```python
from build123d import *

# Parameters (mm, degrees)
SKETCH_1_R      = 2
SKETCH_1_R_2    = 1
EXTRUDE_1_DEPTH = 2
FILLET_1_R      = 2


with BuildPart() as part:
    # 草图1 → 凸台-拉伸1 (new body)
    with BuildSketch(Plane.XY):
        with BuildLine():
            Line((41.276428571, -8.854285714), (-42.723571429, -8.854285714))
            Line((-42.723571429, -8.854285714), (-42.723571429, -21.854285714))
            Line((-42.723571429, -21.854285714), (-54.723571429, -21.854285714))
            Line((-54.723571429, -21.854285714), (-54.723571429, 22.145714286))
            Line((-54.723571429, 22.145714286), (-42.723571429, 22.145714286))
            Line((-42.723571429, 22.145714286), (-42.723571429, 9.145714286))
            Line((-42.723571429, 9.145714286), (41.276428571, 9.145714286))
            ThreePointArc((41.276428571, 9.145714286), (50.276428571, 0.145714286), (41.276428571, -8.854285714))
        make_face()
        with Locations((1.276428571, 0.145714286)):
            Circle(SKETCH_1_R, mode=Mode.SUBTRACT)
        with Locations((-48.723571429, 16.645714286)):
            Circle(SKETCH_1_R, mode=Mode.SUBTRACT)
        with Locations((-48.723571429, -16.354285714)):
            Circle(SKETCH_1_R, mode=Mode.SUBTRACT)
        with Locations((41.276428571, 6.145714286)):
            Circle(SKETCH_1_R_2, mode=Mode.SUBTRACT)
        with Locations((47.276428571, 0.145714286)):
            Circle(SKETCH_1_R_2, mode=Mode.SUBTRACT)
        with Locations((41.276428571, -5.854285714)):
            Circle(SKETCH_1_R_2, mode=Mode.SUBTRACT)
        with Locations((35.276428571, 0.145714286)):
            Circle(SKETCH_1_R_2, mode=Mode.SUBTRACT)
    extrude(amount=EXTRUDE_1_DEPTH)

    # 圆角1
    fillet_1_edges = [part.edges().sort_by_distance(p)[0] for p in [
        (-42.723571429, -8.854285714, 1),
        (-42.723571429, -21.854285714, 1),
        (-54.723571429, -21.854285714, 1),
        (-54.723571429, 22.145714286, 1),
        (-42.723571429, 22.145714286, 1),
        (-42.723571429, 9.145714286, 1),
    ]]
    fillet(fillet_1_edges, radius=FILLET_1_R)


solid = part.part
```
Can you work these out from the model? Positions are in its coordinate system, mm. A direction names the side the tool comes from. Round coordinates to 2 decimals unless told otherwise and drop trailing zeros. Loops run counter-clockwise (first coordinate to the right, second up) from the corner with the lowest first, then second, coordinate; pieces in that order, holes last.
Item 1: Which directions (+Z, -Z, +X, -X, +Y, -Y) give clear straight access to the entire face, cutting with the end or side of a thin tool? Please do faces 5 (the cylindrical face through (-42.12, -9.42, 1.01)), 6 (the flat face through (0, 9.146, 1)).
Item 2: Suppose I cut it at B-B, the plane x = 2. Write out the boundary of the cut face in (y, z), then the cut area to 3 significant figures.
Item 3: Please list where these lines run through material, in increasing order: L1, parallel to X at y = 0, z = 1.6; L2, parallel to X at y = 1, z = 1.65; L3, parallel to Y at x = -6.5, z = 0.9.
Item 4: Will this pin go through, and if not, where does the flat tip stop? pin 1 Ø1 at (x, z) = (-6.5, 1) entering from -Y.
Item 5: Suppose I cut it at C-C, the plane x = 23.5. Write out the boundary of the cut face in (y, z), then the cut area to 3 significant figures.
Item 6: Suppose I cut it at D-D, the plane y = 13. Write out the boundary of the cut face in (x, z).
Item 7: If we mould it in two halves opening along Y, with no side actions, what happens to faces 1 (the flat face through (-13, 0, 2)), 2 (the cylindrical face through (-43.29, 21.54, 1.01)), 3 (the cylindrical face through (42.23, 6.45, 0.99)), 4 (the flat face through (1, -8.854, 1))? For each: +Y half, -Y half, draft (parallel to the pull), parting line (faces both ways), or undercut.
Item 8: Suppose I cut it at A-A, the plane z = 1.1. Write out the boundary of the cut face in (x, y).
Reported:
1. face 5: +Z, -Z, +X, -Y
1. face 6: +Z, -Z, +X, +Y
2. outline: (-8.85, 0) - (-1.72, 0) - (-1.72, 2) - (-8.85, 2) - close; (2.01, 0) - (9.15, 0) - (9.15, 2) - (2.01, 2) - close
2. area: 28.5 mm2
3. L1: x = -54.72 to -0.72, 3.27 to 34.29, 36.27 to 46.29, 48.27 to 50.28
3. L2: x = -54.72 to -0.53, 3.08 to 34.76, 35.8 to 46.76, 47.8 to 50.24
3. L3: y = -8.85 to 9.15
4. pin 1: stops at y = -8.85
5. outline: (-8.85, 0) - (9.15, 0) - (9.15, 2) - (-8.85, 2) - close
5. area: 36.0 mm2
6. outline: (-54.72, 0) - (-42.72, 0) - (-42.72, 2) - (-54.72, 2) - close
7. face 1: draft
7. face 2: +Y half
7. face 3: undercut
7. face 4: -Y half
8. outline: (-54.72, -19.85) arc R2 ccw to (-52.72, -21.85) - (-44.72, -21.85) arc R2 ccw to (-42.72, -19.85) - (-42.72, -10.85) arc R2 cw to (-40.72, -8.85) - (41.28, -8.85) arc R9 ccw to (41.28, 9.15) - (-40.72, 9.15) arc R2 cw to (-42.72, 11.15) - (-42.72, 20.15) arc R2 ccw to (-44.72, 22.15) - (-52.72, 22.15) arc R2 ccw to (-54.72, 20.15) - close; hole circle Ø4 at (-48.72, -16.35); hole circle Ø4 at (-48.72, 16.65); hole circle Ø4 at (1.28, 0.15); hole circle Ø2 at (35.28, 0.15); hole circle Ø2 at (41.28, -5.85); hole circle Ø2 at (41.28, 6.15); hole circle Ø2 at (47.28, 0.15)
